Build history of the part. All positions in model axes, mm. Round coordinates to 2 decimals unless told otherwise and drop trailing zeros. Write each loop counter-clockwise with the first axis right and the second up, starting at its lowest first coordinate (ties: lowest second). Pieces come first, ordered by that corner, then holes. Notation, with made-up numbers: M 85,27.25 L 111,27.25 A26 ccw 111,52.25 Z; hole C 2.5,23 d2. An arc over 180 degrees is marked long. Write item = value, one per line. Start each with the question number.
Q1. Band-saw the part on A-A on y = 0. Write the cut outline in (x, z).
Q2. Band-saw the part on C-C on z = 0. Write the cut outline in (x, y).
Q3. Band-saw the part on B-B on x = 7.15. Write the cut outline in (y, z), plus the area to 3 significant figures.
Q4. Pull direction Z, two halves, no side cores. Call faces 1 (the flat face through (7, -3.5, 1)), 2 (the cylindrical face through (6.5, 0.1, 40.5)), 3 (the cylindrical face through (6.52, 1.03, 35.65)): released by +Z, released by -Z, zero draft, split by the parting line, or undercut.
Q5. Drop flat-ended pins along their axis: P1, Ø2.5, axis at y = 0, z = 0, coming from the -X side; P2, Ø1.5, axis at x = 5.5, y = -1.5, coming from the +Z side. Give the stop position or say it passes through.
Q6. Probe L1, parallel to Z at x = 5.95, y = 0; L2, parallel to Y at x = 5.5, z = -37; L3, parallel to Z at x = 7.2, y = 1. List the from-to ranges inside material, lowest first.
Autodesk Inventor part; units mm, degrees
ref_plane "YZ Plane" through (0, 0, 0) normal (1, 0, 0) x (0, 1, 0)
ref_plane "XZ Plane" through (0, 0, 0) normal (0, 1, 0) x (-1, 0, 0)
ref_plane "XY Plane" through (0, 0, 0) normal (0, 0, 1) x (1, 0, 0)
sketch "Sketch1" plane through (0, 0, 0) normal (1, 0, 0) x (0, 1, 0)
  line L0 (0, 37) -> (0, -37) construction
  line L1 (-3.5, 37) -> (-3.5, -37)
  line L2 (3.5, -37) -> (3.5, 37)
  arc A0 (3.5, 37) -> (-3.5, 37) centre (0, 37) ccw
  arc A1 (-3.5, -37) -> (3.5, -37) centre (0, -37) ccw
  circle A2 centre (0, -37) radius 1.5
  circle A3 centre (0, 0) radius 1.5
  circle A4 centre (0, 37) radius 1.5
  point P0 (0, 40.5)
  point P1 (0, -40.5)
  dimension "d14" = 7
  dimension "d15" = 81
  dimension "d16" = 3
extrude "Extrusión3" add sketch "Sketch1" along normal mid plane 16 contours A0 L2 A1 L1 | A2 | A3 | A4
extrude "Extrusión4" cut sketch "Sketch1" along normal mid plane 10 contours A0 L2 A1 L1 | A3
sketch "Boceto2" plane through (-8, 0, 0) normal (-1, 0, 0) x (0, 0, 1)
  circle A0 centre (37, 0) radius 1.5
  circle A1 centre (-37, 0) radius 1.5
  point P0 (0, 0)
  point P1 (0, 0)
hole "Agujero1" at (-8, 0, 37) at (-8, 0, -37) at (-8, 0, 0) direction (1, 0, 0) diameter 3.4 end through all
split "Dividir1" plane through (0, 0, 0) removes the side toward (-1, 0, 0)
sketch "Boceto3" plane through (-5, 0, 0) normal (1, 0, 0) x (0, 0, -1)
  circle A0 centre (0, 0) radius 1.7
  circle A1 centre (37, 0) radius 1.7
  circle A2 centre (-37, 0) radius 1.7
  arc A3 (37, -3.5) -> (37, 3.5) centre (37, 0) ccw
  line L0 (37, 3.5) -> (-37, 3.5)
  arc A4 (-37, 3.5) -> (-37, -3.5) centre (-37, 0) ccw
  line L1 (-37, -3.5) -> (37, -3.5)
extrude "Extrusión5" cut sketch "Boceto3" against normal blind 10 contours A0 | A1 | A2 | L1 A4 L0 A3
equation "\"d19\" = Dedos"
equation "\"Dedos\" = 10"
properties part number "Corredera I"
Conclusion:
q1.outline = M 5,-40.5 L 8,-40.5 L 8,-38.7 L 5,-38.7 Z; M 5,-35.3 L 8,-35.3 L 8,-1.7 L 5,-1.7 Z; M 5,1.7 L 8,1.7 L 8,35.3 L 5,35.3 Z; M 5,38.7 L 8,38.7 L 8,40.5 L 5,40.5 Z
q2.outline = M 5,-3.5 L 8,-3.5 L 8,-1.7 L 5,-1.7 Z; M 5,1.7 L 8,1.7 L 8,3.5 L 5,3.5 Z
q3.outline = M -3.5,-37 A3.5 ccw 3.5,-37 L 3.5,37 A3.5 ccw -3.5,37 Z; hole C 0,-37 d3.4; hole C 0,0 d3.4; hole C 0,37 d3.4
q3.area = 529 mm^2
q4.face_1 = zero draft
q4.face_2 = released by +Z
q4.face_3 = undercut
q5.P1 = through
q5.P2 = 40.42
q6.L1 = -40.5 to -38.7, -35.3 to -1.7, 1.7 to 35.3, 38.7 to 40.5
q6.L2 = -3.5 to -1.7, 1.7 to 3.5
q6.L3 = -40.35 to -38.37, -35.63 to -1.37, 1.37 to 35.63, 38.37 to 40.35
